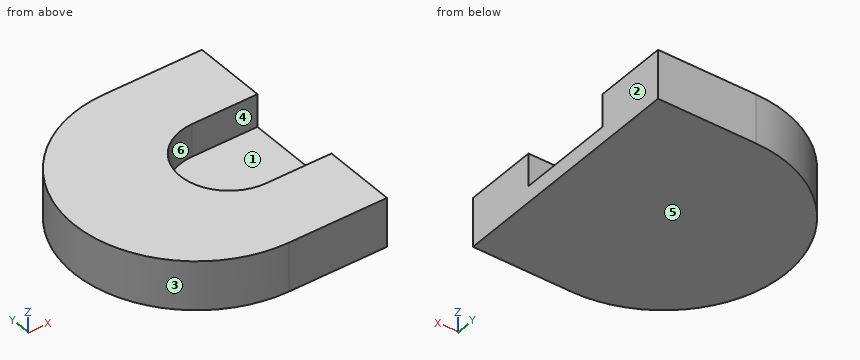
from build123d import *

# Parameters (mm, degrees)
EXTRUDE_1_DEPTH     = 3
CUT_EXTRUDE_1_DEPTH = 2


with BuildPart() as part:
    # Эскиз1 → Бобышка-Вытянуть1 (new body)
    with BuildSketch(Plane.XY):
        with BuildLine():
            Line((0, 7.5), (6, 7.5))
            Line((6, 7.5), (6, -7.5))
            Line((6, -7.5), (0, -7.5))
            ThreePointArc((0, -7.5), (-7.5, 0), (0, 7.5))
        make_face()
    extrude(amount=EXTRUDE_1_DEPTH)

    # Эскиз2 → Вырез-Вытянуть1 (cut)
    with BuildSketch(Plane.XY.offset(3)):
        with BuildLine():
            Line((6, -3), (2, -3))
            ThreePointArc((2, -3), (-1, 0), (2, 3))
            Line((2, 3), (6, 3))
            ThreePointArc((6, 3), (9, 0), (6, -3))
        make_face()
    extrude(amount=-CUT_EXTRUDE_1_DEPTH, mode=Mode.SUBTRACT)


solid = part.part
Source: CAD feature listing. Evaluate the final solid. Frame: model axes, mm. Face numbers are marked on the shaded views. A direction names the side the tool comes from. Coordinates: 2 decimals unless noted, no trailing zeros. Loops run counter-clockwise (first coordinate to the right, second up) from the corner with the lowest first, then second, coordinate; pieces in that order, holes last. Notation, with made-up numbers: (-23.75, 75.25) -> (11.25, 75.25) arc R24 ccw to (11.25, 102.25) -> close; hole circle Ø8 at (-6, -28). An arc over 180 degrees is marked (long way). Answer in a Markdown table with one row per item. Add a question column.
Q1. Section B-B on x = -4.5. Return the cut outline in (y, z).
Q2. Pull-direction query (Y, two-part tool) for the marked faces 1, 2, 3 and 4; classes: pulls with the +Y half, pulls with the -Y half, needs draft (parallel to the pull), parting line crosses it, or undercut.
Q3. Section D-D on x = 1.75. Return the cut outline in (y, z).
Q4. Reachability of the marked faces 5 and 6 from +Z, -Z, +X, -X, +Y, -Y: full face, straight path, thin tool, end or side. Return the list, or none.
Q5. Section A-A on y = 0. Return the cut outline in (x, z), and give its area (3 significant figures).
Q6. Ray query, line 1 along Y through (x, z) = (2.25, 1.75); line 2 along Y through (x, z) = (0.75, 1.05); line 3 along X through (y, z) = (0, 2.45). Return the intervals inside material, ascending.
Q7. Section C-C on z = 0.5. Return the cut outline in (x, y), and give its area (3 significant figures).
Q8. Contact query for a flat-ended pin moving along its axis: pin 1 Ø1.5 at (x, z) = (-5.5, 1) entering from +Y. Output: stop coordinate, or through.
Computed values:
| question | item | result |
|---|---|---|
| 1 | outline | (-6, 0) -> (6, 0) -> (6, 3) -> (-6, 3) -> close |
| 2 | face 1 | undercut |
| 2 | face 2 | needs draft |
| 2 | face 3 | parting line crosses it |
| 2 | face 4 | undercut |
| 3 | outline | (-7.5, 0) -> (7.5, 0) -> (7.5, 3) -> (2.99, 3) -> (2.99, 1) -> (-2.99, 1) -> (-2.99, 3) -> (-7.5, 3) -> close |
| 4 | face 5 | -Z, +X, -X, +Y, -Y |
| 4 | face 6 | +Z, +X |
| 5 | outline | (-7.5, 0) -> (6, 0) -> (6, 1) -> (-1, 1) -> (-1, 3) -> (-7.5, 3) -> close |
| 5 | area | 26.5 mm^2 |
| 6 | line 1 | y = -7.5 to -3, 3 to 7.5 |
| 6 | line 2 | y = -7.5 to -2.73, 2.73 to 7.5 |
| 6 | line 3 | x = -7.5 to -1 |
| 7 | outline | (0, -7.5) -> (6, -7.5) -> (6, 7.5) -> (0, 7.5) arc R7.5 ccw to start |
| 7 | area | 178 mm^2 |
| 8 | pin 1 | stops at y = 5.8 |
